The figure shows three views and two pictorial views of one solid part (mm, origin at its lowest corner). Answer the questions. Give positions to 0.01 mm unless a question says otherwise; leave off trailing zeros. Order: outer loops, then holes, each group sorted by start corner. A loop starts at its lowest first (then second) coordinate and runs counter-clockwise, first axis right, second up. Notation, with made-up numbers: M -12,54 L 34,54 A23 ccw 34,74 Z; hole C 79,28 d9. An arc over 180 degrees is marked long. Answer as a JSON object with one key per item and string values. Group by question number.
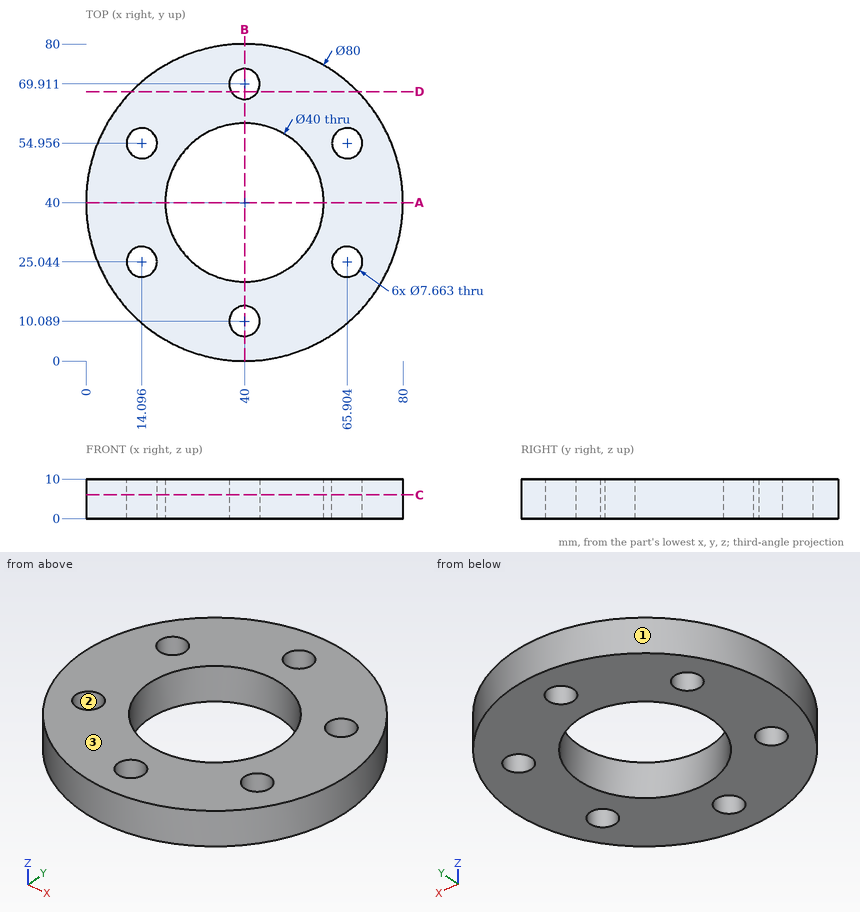
Item 1: Section D-D (y = 68) is taken. Determine the outline of the cut face in (x, z) (1 decimal).
Item 2: Section C-C (z = 6) is taken. Determine the outline of the cut face in (x, y) (1 decimal), and give its area (3 significant figures).
Item 3: Determine the mould class of the marked faces 1, 2 and 3 for opening direction Y: released by +Y, released by -Y, zero draft, split by the parting line, or undercut.
Item 4: Flat-ended cylindrical pins translate along their axes: P1, Ø1.5, axis at x = 34, z = 2, coming from the -Y side; P2, Ø1.5, axis at x = 41.5, z = 2.5, coming from the -Y side; P3, Ø5, axis at x = 42, z = 7, coming from the +Y side. Find the tip coordinate at first contact, or state that the pin passes through.
Item 5: Consider probe 1 along Y at (x, z) = (40, 7.25); probe 2 along X at (y, z) = (54, 1) (1 decimal); probe 3 along X at (y, z) = (25, 3) (1 decimal). Determine where each line is inside the solid, lowest interval first. Write a range as from..to.
Item 6: Section B-B (x = 40) is taken. Determine the outline of the cut face in (y, z), and give its area (3 significant figures).
Item 7: Section A-A (y = 40) is taken. Determine the outline of the cut face in (x, z), and give its area (3 significant figures).
Values found:
{
 "1": {"outline": "M 11.4,0 L 36.7,0 L 36.7,10 L 11.4,10 Z; M 43.3,0 L 68.6,0 L 68.6,10 L 43.3,10 Z"},
 "2": {"outline": "C 40,40 d80; hole C 14.1,25 d7.7; hole C 14.1,55 d7.7; hole C 40,40 d40; hole C 40,10.1 d7.7; hole C 40,69.9 d7.7; hole C 65.9,25 d7.7; hole C 65.9,55 d7.7", "area": "3,490 mm^2"},
 "3": {"face 1": "split by the parting line", "face 2": "undercut", "face 3": "zero draft"},
 "4": {"P1": "stops at y = 0.35", "P2": "stops at y = 0.01", "P3": "stops at y = 80"},
 "5": {"probe 1": "y = 0..6.26, 13.92..20, 60..66.08, 73.74..80", "probe 2": "x = 2.5..10.4, 17.8..25.7, 54.3..62.2, 69.6..77.5", "probe 3": "x = 2.9..10.3, 17.9..26.8, 53.2..62.1, 69.7..77.1"},
 "6": {"outline": "M 0,0 L 6.26,0 L 6.26,10 L 0,10 Z; M 13.92,0 L 20,0 L 20,10 L 13.92,10 Z; M 60,0 L 66.08,0 L 66.08,10 L 60,10 Z; M 73.74,0 L 80,0 L 80,10 L 73.74,10 Z", "area": "247 mm^2"},
 "7": {"outline": "M 0,0 L 20,0 L 20,10 L 0,10 Z; M 60,0 L 80,0 L 80,10 L 60,10 Z", "area": "400 mm^2"}
}
